Build history of the part. All positions in model axes, mm. A direction names the side the tool comes from. Coordinates: 2 decimals unless noted, no trailing zeros. Write each loop counter-clockwise with the first axis right and the second up, starting at its lowest first coordinate (ties: lowest second). Pieces come first, ordered by that corner, then holes.
Autodesk Inventor part; units mm, degrees
ref_plane "YZ Plane" through (0, 0, 0) normal (1, 0, 0) x (0, 1, 0)
ref_plane "XZ Plane" through (0, 0, 0) normal (0, 1, 0) x (-1, 0, 0)
ref_plane "XY Plane" through (0, 0, 0) normal (0, 0, 1) x (1, 0, 0)
sketch "Sketch1" plane through (0, 0, 0) normal (0, 0, 1) x (1, 0, 0)
  line L0 (-173, 120) -> (173, 120)
  line L1 (173, 120) -> (173, -120)
  line L2 (173, -120) -> (-173, -120)
  line L3 (-173, -120) -> (-173, 120)
  point P0 (0, 0)
  dimension "d0" = 173
  dimension "d1" = 240
  dimension "d2" = 346
  dimension "d3" = 120
extrude "Plade tykkelse" add sketch "Sketch1" along normal blind 12
sketch "Sketch2" plane through (0, 0, 12) normal (0, 0, 1) x (1, 0, 0)
  line L0 (5, 88) -> (-145, 88)
  line L1 (5, 88) -> (5, 100)
  line L2 (-145, 100) -> (5, 100)
  line L3 (-145, 88) -> (-145, 100)
  line L4 (5, -100) -> (-145, -100)
  line L5 (5, -100) -> (5, -88)
  line L6 (-145, -88) -> (5, -88)
  line L7 (-145, -100) -> (-145, -88)
  circle A0 centre (-115, 109) radius 3
  circle A1 centre (103, 109) radius 3
  circle A2 centre (-115, -109) radius 3
  circle A3 centre (103, -109) radius 3
  circle A4 centre (-157, 65) radius 6
  circle A5 centre (-157, 0) radius 7
  circle A6 centre (-157, -65) radius 6
  point P0 (0, 0)
  dimension "d22" = 6
  dimension "d23" = 6
  dimension "d24" = 6
  dimension "d25" = 6
  dimension "d26" = 218
  dimension "d27" = 218
  dimension "d28" = 218
  dimension "d29" = 218
  dimension "d36" = 12
  dimension "d37" = 14
  dimension "d38" = 12
  dimension "d39" = 130
  dimension "d40" = 65
  dimension "d41" = 157
  dimension "d42" = 157
  dimension "d43" = 157
  dimension "d44" = 0
  dimension "d45" = 109
  dimension "d46" = 109
  dimension "d64" = 115
  dimension "d65" = 115
extrude "Monteringshuller & -udskæringer" cut sketch "Sketch2" against normal blind 14 contours A0 | A1 | A2 | A3 | A4 | A5 | A6
sketch "Sketch3" plane through (0, 0, 12) normal (0, 0, 1) x (1, 0, 0)
  circle A0 centre (103, -109) radius 3
  line L0 (-173, -120) -> (173, -120)
  line L1 (173, -120) -> (173, 120)
  line L2 (173, 120) -> (111, 120)
  line L3 (111, 120) -> (111, -120)
  line L4 (111, -120) -> (173, -120)
  line L5 (173, -120) -> (173, 120)
  point P0 (0, 0)
  dimension "d47" = 8
extrude "Sidste længde tilpasning" cut sketch "Sketch3" against normal blind 16 contours L3 L2 L1 L0
sketch "Sketch5" plane through (0, 0, 12) normal (0, 0, 1) x (1, 0, 0)
  line L0 (111, 120) -> (-173, 120) construction
  line L1 (-173, 120) -> (-173, -120) construction
  line L2 (-173, -120) -> (111, -120) construction
  circle A0 centre (-157, 0) radius 7 construction
  circle A1 centre (-157, 65) radius 6 construction
  circle A2 centre (-115, -109) radius 3 construction
  circle A3 centre (-115, 109) radius 3 construction
  circle A4 centre (103, 109) radius 3 construction
  circle A5 centre (103, -109) radius 3 construction
  circle A6 centre (-157, -65) radius 6 construction
  line L3 (-173, -120) -> (-173, 120)
  line L4 (-173, -120) -> (-125, -120)
  line L5 (-125, -120) -> (-125, -85)
  line L6 (-125, -85) -> (-173, -85)
  line L7 (-173, -85) -> (-173, -120)
  line L8 (-173, 120) -> (-128, 120)
  line L9 (-128, 120) -> (-128, 85)
  line L10 (-128, 85) -> (-173, 85)
  line L11 (-173, 85) -> (-173, 120)
  line L12 (111, -120) -> (111, 120)
  point P0 (0, 0)
  dimension "d58" = 48
  dimension "d59" = 35
  dimension "d60" = 45
  dimension "d61" = 35
extrude "CutOff" cut sketch "Sketch5" against normal up to surface (12 mm away)
equation "\"d23\" = d22"
equation "\"d24\" = d22"
equation "\"d25\" = d22"
equation "\"d26\" = d29"
equation "\"d27\" = d28"
properties part number "Byggeplade Holder" material "Wood (Cherry)"
1. 3-axis set-ups, long thin cutter, end or side, ignore diameter. For faces 5 (the face through (-125, -103, 6)), 6 (the face through (-150, 85, 6)), 7 (the face through (100.6, -110.8, 6.1)): which of +Z, -Z, +X, -X, +Y, -Y reach the whole face in a straight line?
Computed values:
face 5: +Z, -Z, -X, -Y
face 6: +Z, -Z, -X, +Y
face 7: +Z, -Z
2. Mould opens along Y. For faces 1 (the face through (-149, -85, 6)), 2 (the face through (-163, -65, 6)), 3 (the face through (-128, 103, 6)), 4 (the face through (-10, 120, 6)) say: +Y half, -Y half, draft (parallel to the pull), parting line (faces both ways), or undercut.
Computed values:
face 1: -Y half
face 2: undercut
face 3: draft
face 4: +Y half
3. Saw through at B-B on y = 65. List the corners of the cut face in (x, z), plus the area to 3 significant figures.
Computed values:
outline: (-173, 0) - (-163, 0) - (-163, 12) - (-173, 12) - close; (-151, 0) - (111, 0) - (111, 12) - (-151, 12) - close
area: 3,260 mm2
4. Saw through at C-C on x = -157. List the corners of the cut face in (y, z).
Computed values:
outline: (-85, 0) - (-71, 0) - (-71, 12) - (-85, 12) - close; (-59, 0) - (-7, 0) - (-7, 12) - (-59, 12) - close; (7, 0) - (59, 0) - (59, 12) - (7, 12) - close; (71, 0) - (85, 0) - (85, 12) - (71, 12) - close
5. Probe line 1 along Y through (x, z) = (-157, 9); line 2 along Y through (x, z) = (103, 3.5); line 3 along Y through (x, z) = (-117.5, 9.25). List the from-to ranges inside material, lowest first.
Computed values:
line 1: y = -85 to -71, -59 to -7, 7 to 59, 71 to 85
line 2: y = -120 to -112, -106 to 106, 112 to 120
line 3: y = -120 to -110.66, -107.34 to 107.34, 110.66 to 120
6. Saw through at D-D on z = 4.75. List the corners of the cut face in (x, y), plus the area to 3 significant figures.
Computed values:
outline: (-173, -85) - (-125, -85) - (-125, -120) - (111, -120) - (111, 120) - (-128, 120) - (-128, 85) - (-173, 85) - close; hole circle Ø14 at (-157, 0); hole circle Ø12 at (-157, -65); hole circle Ø12 at (-157, 65); hole circle Ø6 at (-115, -109); hole circle Ø6 at (-115, 109); hole circle Ø6 at (103, -109); hole circle Ø6 at (103, 109)
area: 64,400 mm2
7. Saw through at A-A on y = -109. List the corners of the cut face in (x, z).
Computed values:
outline: (-125, 0) - (-118, 0) - (-118, 12) - (-125, 12) - close; (-112, 0) - (100, 0) - (100, 12) - (-112, 12) - close; (106, 0) - (111, 0) - (111, 12) - (106, 12) - close
8. Flat gauge pins, fed straight in: pin 1 (3.5 mm diameter, centred on x = -151, z = 5, fed in from +Y); pin 2 (19 mm diameter, centred on x = -157, y = 65, fed in from +Z). Where does each tip first touch, or does it go through?
Computed values:
pin 1: stops at y = 85
pin 2: stops at z = 12
